Could you check a few things on this model? Use its own coordinates, in mm. Face numbers are marked on the shaded views. A direction names the side the tool comes from. Round coordinates to 2 decimals unless told otherwise and drop trailing zeros. Loops run counter-clockwise (first coordinate to the right, second up) from the corner with the lowest first, then second, coordinate; pieces in that order, holes last. Notation, with made-up numbers: M 64.5,-7.5 L 71.5,-7.5 A29 cw 71.5,22.5 Z; hole C 41,21 d5. An arc over 180 degrees is marked long. One line per item, written item: value. Start each with the question number.
Q1. Imagine slicing it at B-B (z = 0). Please give me the cut outline in (x, y).
Q2. Which directions (+Z, -Z, +X, -X, +Y, -Y) give clear straight access to the entire face, cutting with the end or side of a thin tool? Please do the marked faces 1 and 2.
Q3. Thinking about a two-plate mould opening in X: for the marked faces 3, 4, 5 and 6, which applies, released by +X, released by -X, zero draft, split by the parting line, or undercut?
Q4. Imagine slicing it at A-A (x = 0). Please give me the cut outline in (y, z), then the cut area to 3 significant figures.
Q5. Please list where these lines run through material, in increasing order: line 1 along X through (y, z) = (2.25, -1); line 2 along Z through (x, y) = (18, 3.25); line 3 along Z through (x, y) = (-18.5, 0.5).
Q6. I'm going to push flat-ended pins straight in: pin 1 Ø3 at (x, z) = (-2.5, 12) entering from +Y; pin 2 Ø3 at (x, y) = (24, 3.5) entering from -Z; pin 3 Ø5 at (x, y) = (6, 1.5) entering from +Z. Where does each tip first touch, or does it pass through?
Q7. Imagine slicing it at C-C (y = 5). Give the number of separate pieces and of enclosed holes in the cut face, then the cut area to 3 significant figures.
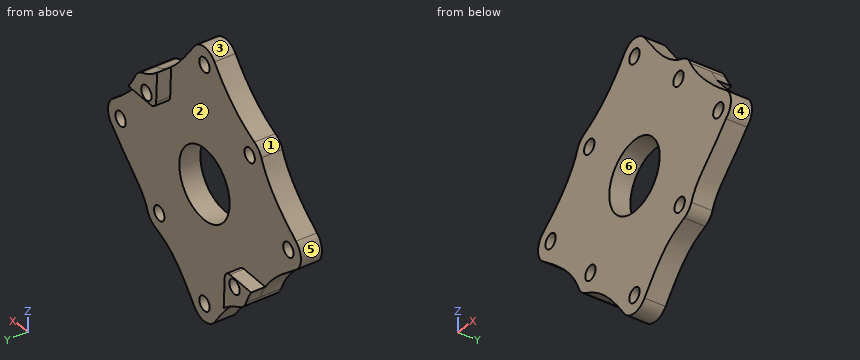
from build123d import *

# Parameters (mm, degrees)
SKETCH2_R           = 2.05
SKETCH2_R_2         = 10
BOSS_EXTRUDE1_DEPTH = 6
SKETCH4_R           = 2.05
BOSS_EXTRUDE2_DEPTH = 4


with BuildPart() as part:
    # Sketch2 → Boss-Extrude1 (new body)
    with BuildSketch(Plane(origin=(0, 0, 0), x_dir=(1, 0, 0), z_dir=(0, 1, 0))):
        with BuildLine():
            ThreePointArc((4, 36.333013665), (0, 38.333013665), (-4, 36.333013665))
            add(Edge.make_bspline(
                [(-19.327049621, 22.155476746), (-12.763587626, 24.730553465), (-8.427522415, 30.156498127), (-4, 36.333013665)],
                knots=[0, 0, 0, 0, 1, 1, 1, 1], degree=3))
            ThreePointArc((-19.327049621, 22.155476746), (-21.03642674, 21.03642674), (-22.155476746, 19.327049621))
            add(Edge.make_bspline(
                [(-36.333013665, 4), (-30.505064465, 8.3709619), (-24.839849632, 12.485009038), (-22.155476746, 19.327049621)],
                knots=[0, 0, 0, 0, 1, 1, 1, 1], degree=3))
            ThreePointArc((-36.333013665, 4), (-38.333013665, 0), (-36.333013665, -4))
            add(Edge.make_bspline(
                [(-36.333013665, -4), (-30.114152071, -8.664146195), (-24.942929086, -13.853392219), (-22.615096154, -19.786669029)],
                knots=[0, 0, 0, 0, 1, 1, 1, 1], degree=3))
            ThreePointArc((-22.615096154, -19.786669029), (-21.496046148, -21.496046148), (-19.786669029, -22.615096154))
            add(Edge.make_bspline(
                [(-19.786669029, -22.615096154), (-12.829111765, -26.205220822), (-8.517950555, -30.309079592), (-4, -36.333013665)],
                knots=[0, 0, 0, 0, 1, 1, 1, 1], degree=3))
            ThreePointArc((-4, -36.333013665), (0, -38.333013665), (4, -36.333013665))
            add(Edge.make_bspline(
                [(4, -36.333013665), (8.986714341, -29.68406121), (12.829629407, -24.073808118), (19.327049621, -22.155476746)],
                knots=[0, 0, 0, 0, 1, 1, 1, 1], degree=3))
            ThreePointArc((19.327049621, -22.155476746), (21.03642674, -21.03642674), (22.155476746, -19.327049621))
            add(Edge.make_bspline(
                [(22.155476746, -19.327049621), (25.018370869, -13.753003663), (31.354300327, -7.734035003), (36.333013665, -4)],
                knots=[0, 0, 0, 0, 1, 1, 1, 1], degree=3))
            ThreePointArc((36.333013665, -4), (38.333013665, 0), (36.333013665, 4))
            add(Edge.make_bspline(
                [(36.333013665, 4), (28.974985707, 12.434827797), (24.849369186, 14.09186156), (22.615096154, 19.786669029)],
                knots=[0, 0, 0, 0, 1, 1, 1, 1], degree=3))
            ThreePointArc((22.615096154, 19.786669029), (21.496046148, 21.496046148), (19.786669029, 22.615096154))
            add(Edge.make_bspline(
                [(4, 36.333013665), (10.902815442, 27.129259742), (13.673195705, 25.013626509), (19.786669029, 22.615096154)],
                knots=[0, 0, 0, 0, 1, 1, 1, 1], degree=3))
        make_face()
        with Locations(Location((0, 33.333013665, 0), (0, 0, 270))):
            Circle(SKETCH2_R, mode=Mode.SUBTRACT)
        with Locations(Location((33.333013665, 0, 0), (0, 0, 270))):
            Circle(SKETCH2_R, mode=Mode.SUBTRACT)
        with Locations(Location((0, -33.333013665, 0), (0, 0, 270))):
            Circle(SKETCH2_R, mode=Mode.SUBTRACT)
        with Locations(Location((-33.333013665, 0, 0), (0, 0, 270))):
            Circle(SKETCH2_R, mode=Mode.SUBTRACT)
        with Locations(Location((0, 0, 0), (0, 0, 270))):
            Circle(SKETCH2_R_2, mode=Mode.SUBTRACT)
        with Locations(Location((-17.500892834, 17.500892834, 0), (0, 0, 270))):
            Circle(SKETCH2_R, mode=Mode.SUBTRACT)
        with Locations(Location((-17.960512242, -17.960512242, 0), (0, 0, 270))):
            Circle(SKETCH2_R, mode=Mode.SUBTRACT)
        with Locations(Location((17.960512242, 17.960512242, 0), (0, 0, 270))):
            Circle(SKETCH2_R, mode=Mode.SUBTRACT)
        with Locations(Location((17.500892834, -17.500892834, 0), (0, 0, 270))):
            Circle(SKETCH2_R, mode=Mode.SUBTRACT)
    extrude(amount=BOSS_EXTRUDE1_DEPTH)

    # Sketch4 → Boss-Extrude2 (add)
    # profile 1 of 2: a face of its own
    with BuildSketch(Plane(origin=(0, 6, 0), x_dir=(1, 0, 0), z_dir=(0, 1, 0))):
        with BuildLine():
            Line((15.707753118, -15.068373573), (24.606369586, -15.466232362))
            add(Edge.make_bspline(
                [(22.155476746, -19.327049621), (22.810102957, -18.052494423), (23.646316442, -16.75467649), (24.606369586, -15.466232362)],
                knots=[0, 0, 0, 0, 0.228658897, 0.228658897, 0.228658897, 0.228658897], degree=3))
            ThreePointArc((22.155476746, -19.327049621), (21.03642674, -21.03642674), (19.327049621, -22.155476746))
            add(Edge.make_bspline(
                [(13.240425147, -25.476068549), (15.048020958, -23.982995667), (17.020234836, -22.836552469), (19.327049621, -22.155476746)],
                knots=[0.644964508, 0.644964508, 0.644964508, 0.644964508, 1, 1, 1, 1], degree=3))
            Line((13.240425147, -25.476068549), (13.620417999, -16.977046436))
            ThreePointArc((13.620417999, -16.977046436), (14.268786465, -15.590408746), (15.707753118, -15.068373573))
        make_face()
        with Locations(Location((17.500892834, -17.500892834, 0), (0, 0, 270))):
            Circle(SKETCH4_R, mode=Mode.SUBTRACT)
    # profile 2 of 2: a face of its own
    with BuildSketch(Plane(origin=(0, 6, 0), x_dir=(1, 0, 0), z_dir=(0, 1, 0))):
        with BuildLine():
            Line((-13.228436316, 25.756908597), (-13.620382808, 16.977307181))
            ThreePointArc((-13.620382808, 16.977307181), (-14.2686581, 15.590625928), (-15.707589672, 15.068494066))
            Line((-15.707589672, 15.068494066), (-24.152657128, 15.445506006))
            add(Edge.make_bspline(
                [(-22.155476746, 19.327049621), (-22.704535018, 17.927587199), (-23.378300091, 16.642253384), (-24.152657128, 15.445506006)],
                knots=[0, 0, 0, 0, 0.204538749, 0.204538749, 0.204538749, 0.204538749], degree=3))
            ThreePointArc((-22.155476746, 19.327049621), (-21.03642674, 21.03642674), (-19.327049621, 22.155476746))
            add(Edge.make_bspline(
                [(-13.228436316, 25.756908597), (-15.059327702, 24.27409121), (-17.060362093, 23.044777893), (-19.327049621, 22.155476746)],
                knots=[0.65465062, 0.65465062, 0.65465062, 0.65465062, 1, 1, 1, 1], degree=3))
        make_face()
        with Locations(Location((-17.500892834, 17.500892834, 0), (0, 0, 270))):
            Circle(SKETCH4_R, mode=Mode.SUBTRACT)
    extrude(amount=BOSS_EXTRUDE2_DEPTH)


solid = part.part
Report:
1. outline: M -38.33,0 L -35.38,0 L -35.38,6 L -38.33,6 Z; M -31.28,0 L -10,0 L -10,6 L -31.28,6 Z; M 10,0 L 31.28,0 L 31.28,6 L 10,6 Z; M 35.38,0 L 38.33,0 L 38.33,6 L 35.38,6 Z
2. face 1: +Z, -X, +Y, -Y
2. face 2: +Y
3. face 3: split by the parting line
3. face 4: released by +X
3. face 5: released by -X
3. face 6: undercut
4. outline: M 0,-38.33 L 6,-38.33 L 6,-35.38 L 0,-35.38 Z; M 0,-31.28 L 6,-31.28 L 6,-10 L 0,-10 Z; M 0,10 L 6,10 L 6,31.28 L 0,31.28 Z; M 0,35.38 L 6,35.38 L 6,38.33 L 0,38.33 Z
4. area: 291 mm²
5. line 1: x = -38.23 to -35.12, -31.54 to -9.95, 9.95 to 31.54, 35.12 to 38.23
5. line 2: z = -23.35 to -20.01, -15.91 to 15.51, 19.49 to 22.61
5. line 3: z = -22.5 to -19.29, -15.71 to 15.98, 19.94 to 23.3
6. pin 1: stops at y = 6
6. pin 2: stops at z = -20.06
6. pin 3: stops at z = 36.9
7. separate pieces: 1
7. enclosed holes: 9
7. area: 2,780 mm²
